Autodesk Inventor part; units mm, degrees
ref_plane "YZ Plane" through (0, 0, 0) normal (1, 0, 0) x (0, 1, 0)
ref_plane "XZ Plane" through (0, 0, 0) normal (0, 1, 0) x (-1, 0, 0)
ref_plane "XY Plane" through (0, 0, 0) normal (0, 0, 1) x (1, 0, 0)
sketch "Sketch1" plane through (0, 0, 0) normal (1, 0, 0) x (0, 1, 0)
  line L0 (0, 0) -> (0, -28.575)
  line L1 (0, -28.575) -> (3.175, -28.575)
  line L2 (3.175, -28.575) -> (3.175, -14.2875)
  line L3 (3.175, -14.2875) -> (9.525, -14.2875)
  line L4 (9.525, -14.2875) -> (9.525, 0)
  line L5 (9.525, 0) -> (0, 0)
  point P0 (0, -14.2875)
  dimension "d0" = 3.175
  dimension "d1" = 9.525
  dimension "d2" = 28.575
extrude "Extrusion1" add sketch "Sketch1" along normal blind 76.2
sketch "Sketch2" plane through (0, 9.525, 0) normal (0, 1, 0) x (1, 0, 0)
  circle A0 centre (15.2237, 21.3995) radius 2.65
  circle A1 centre (40.6237, 21.3995) radius 2.65
  circle A2 centre (66.0237, 21.3995) radius 2.65
  circle A3 centre (55.8475, 8.0482) radius 2.25
  circle A4 centre (6.35, 8.0482) radius 2.25
  line L0 (0, 28.575) -> (0, 14.2875)
  line L1 (0, 14.2875) -> (0, 0)
  line L2 (0, 14.2875) -> (76.2, 14.2875)
  point P0 (0, 21.4313)
  point P1 (0, 7.1438)
  dimension "d5" = 5.3
  dimension "d6" = 25.4
  dimension "d7" = 25.4
  dimension "d8" = 49.4975
  dimension "d9" = 4.5
  dimension "d10" = 13.3513
  dimension "d11" = 8.8737
  dimension "d13" = 7.112
  dimension "d14" = 6.35
extrude "Extrusion2" cut sketch "Sketch2" against normal through all
sketch "Sketch3" plane through (0, 0, -28.575) normal (0, -1, 0) x (1, 0, 0)
  circle A0 centre (55.8475, 20.5268) radius 2.25
  circle A1 centre (55.8475, 20.5268) radius 2.625
  circle A2 centre (6.35, 20.5268) radius 2.25
  circle A3 centre (6.35, 20.5268) radius 2.625
  point P0 (0, 28.575)
  dimension "d17" = 5.25
  dimension "d18" = 5.25
extrude "Extrusion3" cut sketch "Sketch3" against normal blind 5
fillet "Fillet1" radius 6.35 5 edges at (76.2, 4.7625, 0) (38.1, 3.175, -14.2875) (76.2, 1.5875, -28.575) (0, 1.5875, -28.575) (0, 4.7625, 0)
sketch "Sketch4" plane through (0, 9.525, -6.35) normal (0, 1, 0) x (1, 0, 0)
  arc A0 (6.35, 22.225) -> (0, 15.875) centre (6.35, 15.875) ccw
  line L0 (0, 15.875) -> (0, 14.2875)
  line L1 (12.6857, 14.2875) -> (0, 14.2875)
  arc A1 (17.7618, 14.2875) -> (12.6857, 14.2875) centre (15.2237, 15.0495) ccw
  line L2 (38.0857, 14.2875) -> (17.7618, 14.2875)
  arc A2 (43.1618, 14.2875) -> (38.0857, 14.2875) centre (40.6237, 15.0495) ccw
  line L3 (63.4857, 14.2875) -> (43.1618, 14.2875)
  arc A3 (68.5618, 14.2875) -> (63.4857, 14.2875) centre (66.0237, 15.0495) ccw
  line L4 (76.2, 14.2875) -> (68.5618, 14.2875)
  line L5 (76.2, 15.875) -> (76.2, 14.2875)
  arc A4 (76.2, 15.875) -> (69.85, 22.225) centre (69.85, 15.875) ccw
  line L6 (6.35, 22.225) -> (69.85, 22.225)
  circle A5 centre (15.2237, 15.0495) radius 7.112
  circle A6 centre (40.6237, 15.0495) radius 7.112
  circle A7 centre (66.0237, 15.0495) radius 7.112
  point P0 (0, -6.35)
  dimension "d22" = 14.224
  dimension "d23" = 14.224
  dimension "d24" = 14.224
extrude "Extrusion4" cut sketch "Sketch4" against normal up to surface (6.35 mm away) contours A5 L2 A1 L1 | L1 A1 L2 A5 | A7 L3 A3 L4 | L4 A3 L3 A7 | A6 L3 A2 L2 | L2 A2 L3 A6
equation "\"d7\" = d6"
properties part number "DriveMotorMount5"
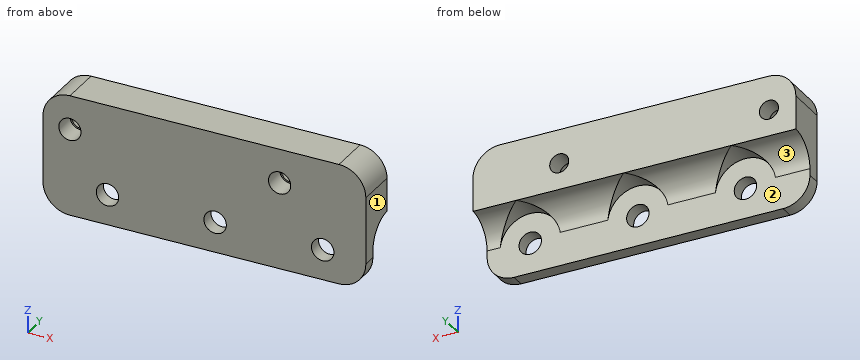
Here's how the part is built. I have some questions about the finished solid (model axes, mm). Face numbers are marked on the shaded views. Round coordinates to 2 decimals unless told otherwise and drop trailing zeros. Loops run counter-clockwise (first coordinate to the right, second up) from the corner with the lowest first, then second, coordinate; pieces in that order, holes last. Notation, with made-up numbers: M -17.75,39 L 36.25,39 A14 ccw 36.25,50 Z; hole C 58.5,-2.75 d3. An arc over 180 degrees is marked long. Write each question's results on one line, items separated by ' | '. Start each with the question number.
(1) Thinking about a two-plate mould opening in X: for the marked faces 1, 2 and 3, which applies, pulls with the +X half, pulls with the -X half, needs draft (parallel to the pull), parting line crosses it, or undercut?
(2) Will these pins go through, and if not, where does the flat tip stop? P1, Ø2, axis at y = 7, z = -16, coming from the +X side; P2, Ø7, axis at x = 40.62, z = -21.4, coming from the +Y side (3 decimals); P3, Ø6, axis at x = 49.5, z = -21, coming from the +Y side.
(3) I want a section at D-D (y = 0.75). State how many separate pieces and enclosed holes the cut face has, then the cut area to 3 significant figures.
(4) I want a section at A-A (z = -8.75). Please give me the cut outline in (x, y) (3 decimals), then the cut area to 3 significant figures.
(5) I want a section at B-B (y = 8.25). Please give me the cut outline in (x, z).
(6) If I drill on probe 1 along X at (y, z) = (3.25, -7.75); probe 2 along X at (y, z) = (3, -8.5); probe 3 along Y at (x, z) = (64, -16.75) (3 decimals), over which ranges is the centre line in solid material (lowest first)? Write a range as from..to.
Solved:
1) face 1: pulls with the +X half | face 2: undercut | face 3: needs draft
2) P1: passes through | P2: stops at y = 3.175 | P3: stops at y = 3.75
3) separate pieces: 1 | enclosed holes: 5 | area: 2,030 mm²
4) outline: M 0,0 L 3.821,0 L 3.821,5 L 4.212,5 L 4.212,9.525 L 0,9.525 Z; M 8.488,5 L 8.879,5 L 8.879,0 L 53.318,0 L 53.318,5 L 53.71,5 L 53.71,9.525 L 8.488,9.525 Z; M 57.985,5 L 58.377,5 L 58.377,0 L 76.2,0 L 76.2,9.525 L 57.985,9.525 Z | area: 637 mm²
5) outline: M 0,-14.42 L 13.87,-14.42 A7.11 cw 16.57,-14.42 L 39.27,-14.42 A7.11 cw 41.97,-14.42 L 64.67,-14.42 A7.11 cw 67.37,-14.42 L 76.2,-14.42 L 76.2,-6.35 A6.35 ccw 69.85,0 L 6.35,0 A6.35 ccw 0,-6.35 Z; hole C 6.35,-8.05 d4.5; hole C 55.85,-8.05 d4.5
6) probe 1: x = 0..3.74, 8.96..53.24, 58.46..76.2 | probe 2: x = 0..3.76, 8.94..53.26, 58.43..76.2 | probe 3: y = 0..3.175
